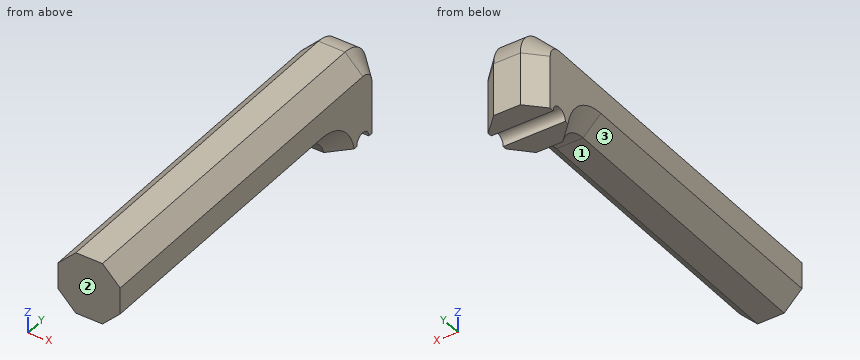
from build123d import *

# Parameters (mm, degrees)
Y_KSEKLIK_EKSTR_ZYON4_DEPTH = 35
RADYUS1_R                   = 17.5
RADYUS2_R                   = 17.5
IZIM4_R                     = 5
KES_EKSTR_ZYON1_DEPTH       = 223.331396793
PAH1_SIZE                   = 10
PAH2_SIZE                   = 10
PAH4_SIZE                   = 10
PAH5_SIZE                   = 10


with BuildPart() as part:
    # Çizim3 → Yükseklik-Ekstrüzyon4 (new body)
    with BuildSketch(Plane(origin=(0, 0, 0), x_dir=(0, 0, -1), z_dir=(1, 0, 0))):
        Polygon((17.5, 182.5), (17.5, 0), (-17.5, 0), (-17.5, 217.5), (30, 217.5), (30, 182.5), align=None)
    extrude(amount=Y_KSEKLIK_EKSTR_ZYON4_DEPTH)

    # Radyus1
    radyus1_edges = [part.edges().sort_by_distance(p)[0] for p in [
        (17.5, 217.5, 17.5),
    ]]
    fillet(radyus1_edges, radius=RADYUS1_R)

    # Radyus2
    # the kernel refuses this fillet: 17.5 mm, written as the material it adds along each edge
    with BuildSketch(Plane(origin=(0, 182.5, -17.5), x_dir=(0, -1, 0), z_dir=(1, 0, 0))) as radyus2_piece_1:
        with BuildLine():
            CenterArc((16.770509831, 17.5), RADYUS2_R, 196.601549599, 73.398450401)
            Line((0, 12.5), (-0.335410197, 12.4))
            ThreePointArc((-0.335410197, 12.4), (-0.35, 6.25), (-0.35, 0))
            Line((-0.35, 0), (0, -0.35))
            Line((0, -0.35), (16.770509831, -0.35))
            Line((16.770509831, -0.35), (16.770509831, 0))
        make_face()
    extrude(amount=35)

    # Çizim4 → Kes-Ekstrüzyon1 (cut, through all)
    with BuildSketch(Plane(origin=(35, 0, 0), x_dir=(0, 0, -1), z_dir=(1, 0, 0))):
        with Locations((30, 200)):
            Circle(IZIM4_R)
    extrude(amount=-KES_EKSTR_ZYON1_DEPTH, mode=Mode.SUBTRACT)

    # Pah1
    pah1_edges = [part.edges().sort_by_distance(p)[0] for p in [
        (0, 100, 17.5),
        (0, 212.374368671, 12.374368671),
        (0, 217.5, -15),
    ]]
    chamfer(pah1_edges, length=PAH1_SIZE)

    # Pah2
    pah2_edges = [part.edges().sort_by_distance(p)[0] for p in [
        (35, 217.5, -15),
        (35, 100, 17.5),
        (35, 212.374368671, 12.374368671),
    ]]
    chamfer(pah2_edges, length=PAH2_SIZE)

    # Pah4
    pah4_edges = [part.edges().sort_by_distance(p)[0] for p in [
        (35, 82.864745084, -17.5),
        (35, 176.1877405, -20.9687848),
    ]]
    chamfer(pah4_edges, length=PAH4_SIZE)

    # Pah5
    pah5_edges = [part.edges().sort_by_distance(p)[0] for p in [
        (0, 176.1877405, -20.9687848),
        (0, 82.864745084, -17.5),
    ]]
    chamfer(pah5_edges, length=PAH5_SIZE)


solid = part.part
Geometry: final body of the model. Coordinates: model frame, mm. Face numbers are marked on the shaded views. A direction names the side the tool comes from. Give positions to 0.01 mm unless a question says otherwise; leave off trailing zeros. Write each loop counter-clockwise with the first axis right and the second up, starting at its lowest first coordinate (ties: lowest second). Pieces come first, ordered by that corner, then holes.
(1) Cut plane A-A, the plane x = 22. Return loops of the section in (y, z).
(2) Ray query, line 1 (Z direction, x = 20.5, y = 36); line 2 (Y direction, x = 32, z = -27.5); line 3 (Y direction, x = 18, z = 1). Return the intervals inside material, ascending.
(3) First-contact query: P1, Ø2, axis at y = 158, z = -14, coming from the +X side; P2, Ø10, axis at y = 76, z = -15.5, coming from the -X side; P3, Ø7.5, axis at x = 17, y = 58, coming from the -Z side. Flat tips, straight axial feed; report the tip coordinate or a pass-through.
(4) Cut plane C-C, the plane x = 32. Return loops of the section in (y, z).
(5) Cut plane B-B, the plane y = 122.5. Return loops of the section in (x, z), then the cut area to 4 significant figures.
(6) Access query for the marked faces 1, 2 and 3. Directions: +Z, -Z, +X, -X, +Y, -Y. A direction counts if a zero-diameter tool reaches every point of the face in a straight line with its end or side. Return the directions, or none.
Values follow:
1. outline: (0, -17.5) - (165.73, -17.5) arc R17.5 cw to (182.5, -30) - (195, -30) arc R5 cw to (205, -30) - (217.5, -30) - (217.5, 0) arc R17.5 ccw to (200, 17.5) - (0, 17.5) - close
2. line 1: z = -17.5 to 17.5
2. line 2: y = 189.05 to 195.67, 204.33 to 210.5
2. line 3: y = 0 to 217.47
3. P1: stops at x = 29.5
3. P2: stops at x = 3
3. P3: stops at z = -17.5
4. outline: (0, -10.5) - (165.73, -10.5) arc R24.5 cw to (189.71, -30) - (195, -30) arc R5 cw to (205, -30) - (210.5, -30) - (210.5, 0) arc R10.5 ccw to (200, 10.5) - (0, 10.5) - close
5. outline: (0, -7.5) - (10, -17.5) - (25, -17.5) - (35, -7.5) - (35, 7.5) - (25, 17.5) - (10, 17.5) - (0, 7.5) - close
5. area: 1,025 mm2
6. face 1: -Z, +X, -X, -Y
6. face 2: +Z, -Z, +X, -X, -Y
6. face 3: -Z, -X, -Y
